The listing builds one solid part. Answer for the finished solid, in the listing's coordinates (mm). Coordinates: 2 decimals unless noted, no trailing zeros. Order: outer loops, then holes, each group sorted by start corner. A loop starts at its lowest first (then second) coordinate and runs counter-clockwise, first axis right, second up. Notation, with made-up numbers: (29.5, 77.25) -> (53.5, 77.25) arc R24 ccw to (53.5, 106.25) -> close; hole circle Ø11 at (-20, 71.5). An arc over 180 degrees is marked (long way). Answer in a Markdown table with one row per item.
```python
from build123d import *

# Parameters (mm, degrees)
BOSS_EXTRUDE1_DEPTH      = 3.175
SKETCH2_R                = 1.5
SKETCH2_R_2              = 2.25
CUT_EXTRUDE1_DEPTH       = 171.725102504
M3X0_5_TAPPED_HOLE1_D    = 2.5
SKETCH5_R                = 1.25
CUT_EXTRUDE2_DEPTH       = 171.725102504
SKETCH6_R                = 1.25
CUT_EXTRUDE3_DEPTH       = 10
M4_CLEARANCE_HOLE1_D     = 4.5
M4_CLEARANCE_HOLE1_DEPTH = 10
M4_CLEARANCE_HOLE1_TIP   = 1.351936393
M3X0_5_TAPPED_HOLE2_D    = 2.5
SKETCH15_W               = 131.4
SKETCH15_H               = 3.175
BOSS_EXTRUDE2_DEPTH      = 5
FILLET1_R                = 5
FILLET2_SIZE             = 5


# Some blends are built 0.0001 mm under size
with BuildPart() as part:
    # Sketch1 → Boss-Extrude1 (new body)
    with BuildSketch(Plane(origin=(0, 0, 0), x_dir=(1, 0, 0), z_dir=(0, 1, 0))):
        Polygon((-110.7, 120.7), (110.7, 120.7), (120.7, 110.7), (120.7, -110.7), (110.7, -120.7), (-110.7, -120.7), (-120.7, -110.7), (-120.7, 110.7), align=None)
    extrude(amount=BOSS_EXTRUDE1_DEPTH)

    # Sketch2 → Cut-Extrude1 (cut, through all)
    with BuildSketch(Plane(origin=(0, 3.175, 0), x_dir=(1, 0, 0), z_dir=(0, 1, 0))):
        with Locations(Location((-51, -40, 0), (0, 0, 270))):
            Circle(SKETCH2_R)
        with Locations(Location((-29, -40, 0), (0, 0, 270))):
            Circle(SKETCH2_R_2)
        with Locations(Location((-51, 40, 0), (0, 0, 270))):
            Circle(SKETCH2_R)
        with Locations(Location((-29, 40, 0), (0, 0, 270))):
            Circle(SKETCH2_R_2)
        with Locations(Location((29, 40, 0), (0, 0, 270))):
            Circle(SKETCH2_R_2)
        with Locations(Location((51, 40, 0), (0, 0, 270))):
            Circle(SKETCH2_R_2)
        with Locations(Location((29, -40, 0), (0, 0, 270))):
            Circle(SKETCH2_R_2)
        with Locations(Location((51, -40, 0), (0, 0, 270))):
            Circle(SKETCH2_R_2)
        with Locations(Location((-3.5, 0, 0), (0, 0, 270))):
            Circle(SKETCH2_R_2)
        with Locations(Location((-13.5, 22, 0), (0, 0, 270))):
            Circle(SKETCH2_R_2)
        with Locations(Location((-13.5, -22, 0), (0, 0, 270))):
            Circle(SKETCH2_R_2)
    extrude(amount=-CUT_EXTRUDE1_DEPTH, mode=Mode.SUBTRACT)

    # M3x0.5 Tapped Hole1 (through all)
    with Locations(Plane(origin=(0, 3.175, 0), x_dir=(-1, 0, 0), z_dir=(0, 1, 0))):
        with Locations((114.5, -104.5), (104.5, -114.5), (-104.5, -114.5), (-114.5, -104.5), (-114.5, 104.5), (-104.5, 114.5), (104.5, 114.5), (114.5, 104.5), (-104.5, 104.5), (-104.5, -104.5), (104.5, -104.5), (104.5, 104.5)):
            Hole(M3X0_5_TAPPED_HOLE1_D / 2)

    # Sketch5 → Cut-Extrude2 (cut, through all)
    with BuildSketch(Plane(origin=(0, 3.175, 0), x_dir=(1, 0, 0), z_dir=(0, 1, 0))):
        with Locations(Location((-55, 95, 0), (0, 0, 270))):
            Circle(SKETCH5_R)
        with Locations(Location((55, 95, 0), (0, 0, 270))):
            Circle(SKETCH5_R)
        with Locations(Location((-55, -95, 0), (0, 0, 270))):
            Circle(SKETCH5_R)
        with Locations(Location((55, -95, 0), (0, 0, 270))):
            Circle(SKETCH5_R)
    extrude(amount=-CUT_EXTRUDE2_DEPTH, mode=Mode.SUBTRACT)

    # Sketch6 → Cut-Extrude3 (cut)
    with BuildSketch(Plane(origin=(0, 3.175, 0), x_dir=(1, 0, 0), z_dir=(0, 1, 0))):
        with Locations(Location((-91.2, -64.7, 0), (0, 0, 270))):
            Circle(SKETCH6_R)
        with Locations(Location((-91.2, -56.7, 0), (0, 0, 270))):
            Circle(SKETCH6_R)
        with Locations(Location((-91.2, -79.7, 0), (0, 0, 270))):
            Circle(SKETCH6_R)
    extrude(amount=-CUT_EXTRUDE3_DEPTH, mode=Mode.SUBTRACT)

    # M4 Clearance Hole1
    with Locations(Plane(origin=(0, 3.175, 0), x_dir=(-1, 0, 0), z_dir=(0, 1, 0))):
        with Locations((51, -40), (51, 40)):
            Hole(M4_CLEARANCE_HOLE1_D / 2, depth=M4_CLEARANCE_HOLE1_DEPTH)
            with Locations((0, 0, -(M4_CLEARANCE_HOLE1_DEPTH + M4_CLEARANCE_HOLE1_TIP / 2))):  # 118° drill point
                Cone(0, M4_CLEARANCE_HOLE1_D / 2, M4_CLEARANCE_HOLE1_TIP, mode=Mode.SUBTRACT)

    # M3x0.5 Tapped Hole2 (through all)
    with Locations(Plane(origin=(0, 3.175, 0), x_dir=(-1, 0, 0), z_dir=(0, 1, 0))):
        with Locations((-55.188488938, -111.84444349), (54.811511062, -111.84444349), (-55.188488938, -116.267236791), (54.811511062, -116.267236791)):
            Hole(M3X0_5_TAPPED_HOLE2_D / 2)

    # Sketch15 → Boss-Extrude2 (add)
    with BuildSketch(Plane(origin=(0, 0, -120.7), x_dir=(-1, 0, 0), z_dir=(0, 0, -1))):
        with Locations((0, 1.5875)):
            Rectangle(SKETCH15_W, SKETCH15_H)
    extrude(amount=BOSS_EXTRUDE2_DEPTH)

    # Fillet1
    fillet1_edges = [part.edges().sort_by_distance(p)[0] for p in [
        (-65.7, 1.5875, -125.7),
    ]]
    fillet(fillet1_edges, radius=FILLET1_R - 0.0001)  # a hair under: the kernel refuses the full size

    # Fillet2
    # a fillet whose section is not a circle: 5 mm, written as the material it takes off along each edge
    with BuildSketch(Plane(origin=(65.7, -12.5, -125.7), x_dir=(-1, 0, 0), z_dir=(0, 1, 0))) as fillet2_piece_1:
        with BuildLine():
            Bezier((FILLET2_SIZE, 0), (0, 0), (0, FILLET2_SIZE), weights=[1, 1, 1])
            Line((0, FILLET2_SIZE), (0, 0))
            Line((0, 0), (FILLET2_SIZE, 0))
        make_face()
    extrude(amount=28.175, mode=Mode.SUBTRACT)


solid = part.part
```
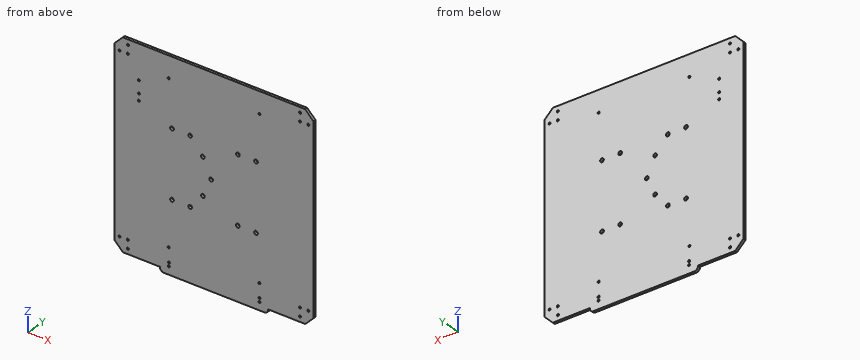
(1) A cutting plane is placed at B-B, the plane y = 1.6. Count the separate pieces of the cut face and the enclosed holes in it, then the cut area to 3 significant figures.
Check values:
| item | result |
|---|---|
| separate pieces | 1 |
| enclosed holes | 34 |
| area | 58,400 mm² |
(2) Find the intervals of material crossed by line 1 along Z through (x, y) = (-104.5, 1.2); line 2 along X through (y, z) = (0.35, -40.5), in increasing order. Write a range as from..to.
Check values:
| item | result |
|---|---|
| line 1 | -120.7..-115.75, -113.25..-105.75, -103.25..103.25, 105.75..113.25, 115.75..120.7 |
| line 2 | -120.7..-53.19, -48.81..-31.19, -26.81..26.81, 31.19..48.81, 53.19..120.7 |
(3) A cutting plane is placed at A-A, the plane x = 92. Determine the outline of the cut face in (y, z) (3 decimals).
Check values:
| item | result |
|---|---|
| outline | (0, -120.7) -> (3.175, -120.7) -> (3.175, 120.7) -> (0, 120.7) -> close |
(4) Flat-ended cylindrical pins translate along their axes: pin 1 (3.5 mm diameter, centred on x = -51, z = -40, fed in from +Y); pin 2 (1 mm diameter, centred on x = -79.5, y = 1.5, fed in from -Z). Find the tip coordinate at first contact, or state that the pin passes through.
Check values:
| item | result |
|---|---|
| pin 1 | through |
| pin 2 | z = -120.7 |
